Job drawing, mm, ordinate dimensions from the low corner. One solid piece. Coordinates: 2 decimals unless noted, no trailing zeros. Write each loop counter-clockwise with the first axis right and the second up, starting at its lowest first coordinate (ties: lowest second). Pieces come first, ordered by that corner, then holes. Notation, with made-up numbers: (-5, -5.75) - (25, -5.75) arc R12 cw to (25, 12.25) - close; hole circle Ø7 at (11.5, -37). An arc over 180 degrees is marked (long way). Put each result on its own line as item: value. Start each with the question number.
1. Saw through at B-B, the plane z = 28.5. Write the cut outline in (x, y).
2. Saw through at A-A, the plane x = 38.1. Write the cut outline in (y, z).
3. Drop a flat-ended pin along its axis: P1, Ø1, axis at y = 4.5, z = 10.5, coming from the -X side. Give the stop position or say it passes through.
4. Pull direction X, two halves, no side cores. Call the marked faces 1, 2 and 3: released by +X, released by -X, zero draft, split by the parting line, or undercut.
5. Saw through at C-C, the plane y = 1.75. Give the number of separate pieces and of enclosed holes in the cut face, plus the area to 3 significant figures.
6. Saw through at D-D, the plane x = 19.05. Write the cut outline in (y, z).
7. Drill centre lines: L1, parallel to X at y = 2, z = 25.4; L2, parallel to Z at x = 19.05, y = 2.75 (1 decimal); L3, parallel to Z at x = 25.4, y = 4.5. Where is each one in solid material? Low to high. Write a range as from..to.
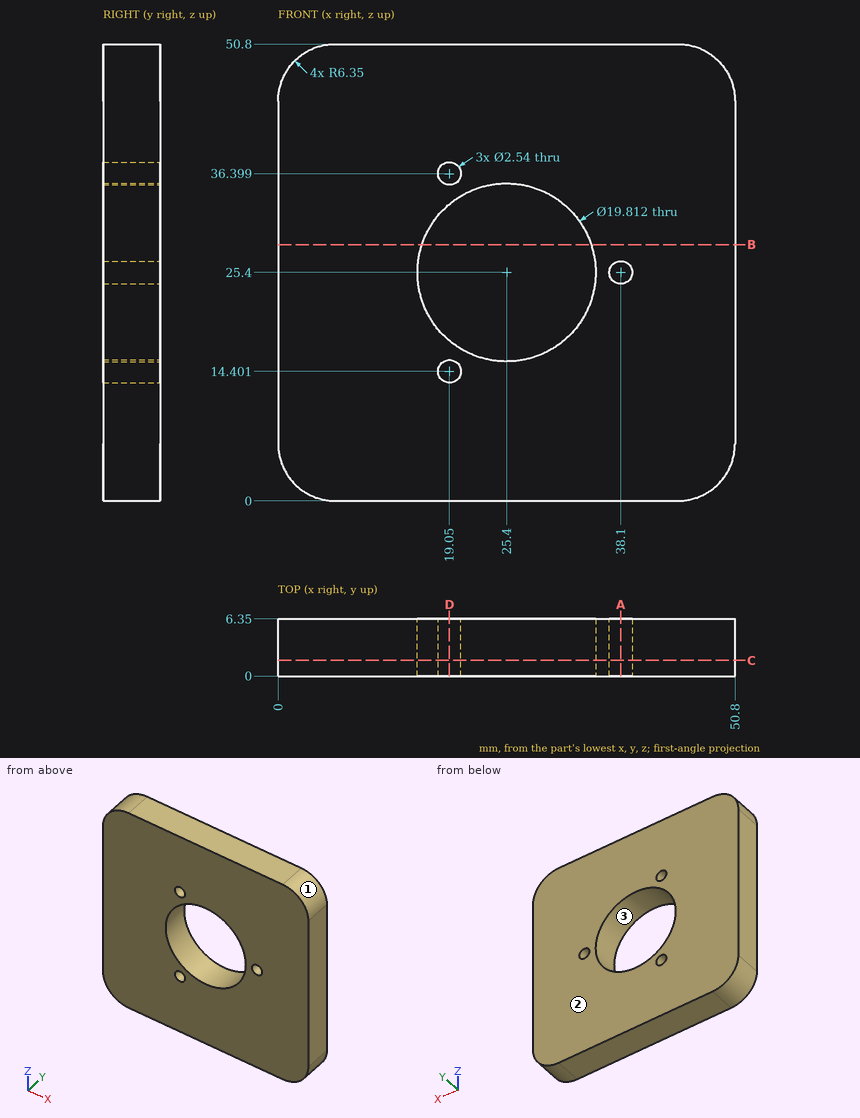
Final values:
1. outline: (0, 0) - (15.99, 0) - (15.99, 6.35) - (0, 6.35) - close; (34.81, 0) - (50.8, 0) - (50.8, 6.35) - (34.81, 6.35) - close
2. outline: (0, 0) - (6.35, 0) - (6.35, 24.13) - (0, 24.13) - close; (0, 26.67) - (6.35, 26.67) - (6.35, 50.8) - (0, 50.8) - close
3. P1: stops at x = 0
4. face 1: released by +X
4. face 2: zero draft
4. face 3: undercut
5. separate pieces: 1
5. enclosed holes: 4
5. area: 2,220 mm²
6. outline: (0, 0) - (6.35, 0) - (6.35, 13.13) - (0, 13.13) - close; (0, 15.67) - (6.35, 15.67) - (6.35, 17.8) - (0, 17.8) - close; (0, 33) - (6.35, 33) - (6.35, 35.13) - (0, 35.13) - close; (0, 37.67) - (6.35, 37.67) - (6.35, 50.8) - (0, 50.8) - close
7. L1: x = 0..15.49, 35.31..36.83, 39.37..50.8
7. L2: z = 0..13.1, 15.7..17.8, 33..35.1, 37.7..50.8
7. L3: z = 0..15.49, 35.31..50.8
